from build123d import *

# Parameters (mm, degrees)
F0_W     = 40.8432
F0_H     = 51.3588
F0_R     = 1.5875
F1_DEPTH = 1.5875
F3_DEPTH = 0.396875


with BuildPart() as f1:
    # F0 (on Top) → F1 (new body)
    with BuildSketch(Plane.XY):
        Rectangle(F0_W, F0_H)
        with Locations((-17.8181, -21.5519)):
            Circle(F0_R, mode=Mode.SUBTRACT)
        with Locations((-9.7409, 23.0759)):
            Circle(F0_R, mode=Mode.SUBTRACT)
        with Locations((0.1143, 4.0513)):
            Circle(F0_R, mode=Mode.SUBTRACT)
        with Locations((9.7409, 23.0759)):
            Circle(F0_R, mode=Mode.SUBTRACT)
    extrude(amount=F1_DEPTH)

    # F2 (on face) → F3 (cut)
    with BuildSketch(Plane.XY.offset(1.5875)):
        Polygon((4.5466, 25.6794), (-4.9784, 25.6794), (-12.7, 19.3294), (-12.7, -2.8956), (12.7, -2.8956), (12.7, 19.3294), align=None)
    extrude(amount=-F3_DEPTH, mode=Mode.SUBTRACT)


solid = f1.part
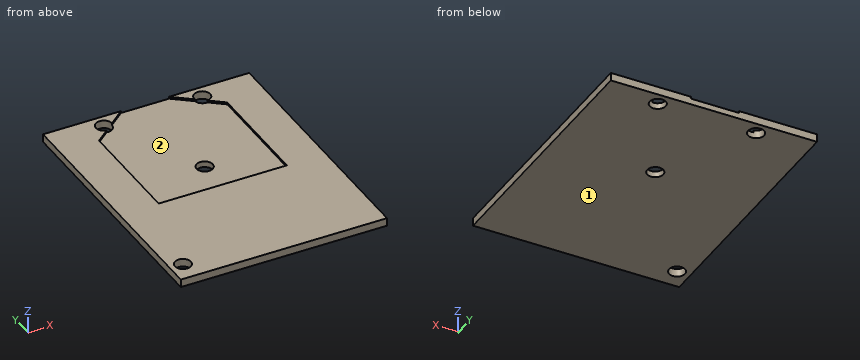
CAD build for the part. Positions are in the model's coordinates, mm. Face numbers are marked on the shaded views. Round coordinates to 2 decimals unless told otherwise and drop trailing zeros. Order: outer loops, then holes, each group sorted by start corner. A loop starts at its lowest first (then second) coordinate and runs counter-clockwise, first axis right, second up. Notation, with made-up numbers: (-24.75, 27) -> (-0.75, 27) arc R21 ccw to (-0.75, 38) -> close; hole circle Ø5 at (30, 75). An arc over 180 degrees is marked (long way). Write each question's results on one line, items separated by ' | '.
1. Flat gauge pins, fed straight in: P1, Ø3, axis at x = -9.74, y = 23.08, coming from the +Z side; P2, Ø20.5, axis at x = 2, y = 11.5, coming from the +Z side. Where does each tip first touch, or does it go through?
Findings below:
P1: passes through | P2: stops at z = 1.19
2. Cut at D-D (x = 3.5). Give the cut face in (y, z), plus the area to 3 significant figures.
Findings below:
outline: (-25.68, 0) -> (25.68, 0) -> (25.68, 1.19) -> (-2.9, 1.19) -> (-2.9, 1.59) -> (-25.68, 1.59) -> close | area: 70.2 mm²
3. Wall check: line 1 along Z through (x, y) = (2.5, 9.5); line 2 along Y through (x, z) = (9.5, 1.4); line 3 along Y through (x, z) = (-16.5, 1.2). Give the ranges that are in metal, low to high. Write a range as [from, to].
Findings below:
line 1: z = [0, 1.19] | line 2: y = [-25.68, -2.9], [24.65, 25.68] | line 3: y = [-25.68, -22.44], [-20.67, 25.68]
4. Cut at A-A (x = -9.5). Give the cut face in (y, z).
Findings below:
outline: (-25.68, 0) -> (21.51, 0) -> (21.51, 1.19) -> (-2.9, 1.19) -> (-2.9, 1.59) -> (-25.68, 1.59) -> close; (24.65, 0) -> (25.68, 0) -> (25.68, 1.59) -> (24.65, 1.59) -> close
5. Cut at B-B (y = 0.5). Give the cut face in (x, z), plus the area to 3 significant figures.
Findings below:
outline: (-20.42, 0) -> (20.42, 0) -> (20.42, 1.59) -> (12.7, 1.59) -> (12.7, 1.19) -> (-12.7, 1.19) -> (-12.7, 1.59) -> (-20.42, 1.59) -> close | area: 54.8 mm²
6. Pull direction X, two halves, no side cores. Call the marked faces 1 and 2: pulls with the +X half, pulls with the -X half, needs draft (parallel to the pull), parting line crosses it, or undercut.
Findings below:
face 1: needs draft | face 2: undercut
7. Cut at C-C (z = 0.55). Give the cut face in (x, y) (1 decimal).
Findings below:
outline: (-20.4, -25.7) -> (20.4, -25.7) -> (20.4, 25.7) -> (-20.4, 25.7) -> close; hole circle Ø3.2 at (-17.8, -21.6); hole circle Ø3.2 at (-9.7, 23.1); hole circle Ø3.2 at (0.1, 4.1); hole circle Ø3.2 at (9.7, 23.1)
